Here's how the part is built. I have some questions about the finished solid (model axes, mm). A direction names the side the tool comes from. Round coordinates to 2 decimals unless told otherwise and drop trailing zeros. Order: outer loops, then holes, each group sorted by start corner. A loop starts at its lowest first (then second) coordinate and runs counter-clockwise, first axis right, second up. Notation, with made-up numbers: M -14.75,81 L 22.25,81 A30 ccw 22.25,112 Z; hole C 80.5,13.5 d10. An arc over 180 degrees is marked long. Write item = value, one per line. Start each with the question number.
Item 1: Please list where these lines run through material, in increasing order: L1, parallel to Z at x = -11.5, y = 9; L2, parallel to Y at x = 3.5, z = 0.65; L3, parallel to Y at x = -2.5, z = -0.55.
Item 2: We'd pull the mould along Z, two halves only. Please class faces 1 (the face through (-0.252, 21.657, -0.852)), 2 (the face through (-0.3, -23, 0.5)), 3 (the face through (0, 0, 1)): pulls with the +Z half, pulls with the -Z half, needs draft (parallel to the pull), parting line crosses it, or undercut.
Item 3: I want a section at B-B, the plane y = -16. List the corners of the cut face in (x, z) for me, plus the area to 3 significant figures.
Item 4: I'm going to push a flat-ended pin straight in: P1, Ø1, axis at x = 8.5, y = -15.5, coming from the -Z side. Where does the tip first touch, or does it pass through?
Item 5: For faces 4 (the face through (18, 0, 0.5)), 5 (the face through (-0.3, 23, 0.5)), which set-ups out of +Z, -Z, +X, -X, +Y, -Y let a thin tool reach every point of the face, with its end or its side?
```python
from build123d import *

# Parameters (mm, degrees)
F0_W     = 36
F0_H     = 46
F1_DEPTH = 1
F2_R     = 0.5
F3_DEPTH = 18


with BuildPart() as f1:
    # F0 (on Top) → F1 (new body)
    with BuildSketch(Plane.XY):
        Rectangle(F0_W, F0_H)
    extrude(amount=F1_DEPTH)

    # F2 (on Right) → F3 (join, symmetric)
    with BuildSketch(Plane.YZ):
        with BuildLine():
            Line((22.966417, 0), (21.345964, 0))
            ThreePointArc((21.345964, 0), (22.15619, -1.575722), (22.966417, 0))
        make_face()
        with Locations((22.15619, -0.874182)):
            Circle(F2_R, mode=Mode.SUBTRACT)
    extrude(amount=F3_DEPTH, both=True)


solid = f1.part
```
Filled in:
q1.L1 = 0 to 1
q1.L2 = -23 to 23
q1.L3 = 21.16 to 21.78, 22.54 to 23.15
q2.face_1 = undercut
q2.face_2 = needs draft
q2.face_3 = pulls with the +Z half
q3.outline = M -18,0 L 18,0 L 18,1 L -18,1 Z
q3.area = 36.0 mm^2
q4.P1 = 0
q5.face_4 = +Z, -Z, +X, +Y, -Y
q5.face_5 = +Z, +X, -X, +Y
